CAD build for the part. Positions are in the model's coordinates, mm. A direction names the side the tool comes from. Round coordinates to 2 decimals unless told otherwise and drop trailing zeros. Loops run counter-clockwise (first coordinate to the right, second up) from the corner with the lowest first, then second, coordinate; pieces in that order, holes last.
Autodesk Inventor part; units mm, degrees
ref_plane "YZ Plane" through (0, 0, 0) normal (1, 0, 0) x (0, 1, 0)
ref_plane "XZ Plane" through (0, 0, 0) normal (0, 1, 0) x (-1, 0, 0)
ref_plane "XY Plane" through (0, 0, 0) normal (0, 0, 1) x (1, 0, 0)
sketch "Sketch1" plane through (0, 0, 0) normal (0, 0, 1) x (1, 0, 0)
  line L0 (-14, 17.1738) -> (14, 17.1738)
  line L1 (14, 17.1738) -> (14, -17.1738)
  line L2 (14, -32.8262) -> (-14, -32.8262)
  line L3 (-14, -32.8262) -> (-14, -17.1738)
  arc A0 (-14, -17.1738) -> (14, -17.1738) centre (0, -32.8262) ccw
  line L4 (-14, -17.1738) -> (-14, 17.1738)
  line L5 (14, -17.1738) -> (14, -32.8262)
  point P0 (0, 0)
  point P1 (0, 17.1738)
  point P2 (14, 0)
  dimension "d0" = 42
  dimension "d1" = 50
  dimension "d4" = 28
extrude "Extrusion1" add sketch "Sketch1" along normal blind 3
sketch "Sketch2" plane through (0, 0, 3) normal (0, 0, 1) x (1, 0, 0)
  line L0 (14, -17.1738) -> (14, 17.1738)
  line L1 (14, 17.1738) -> (-14, 17.1738) construction
  line L2 (-14, 17.1738) -> (-14, -17.1738) construction
  arc A0 (-14, -17.1738) -> (14, -17.1738) centre (0, -32.8262) ccw
  circle A1 centre (0, -32.8262) radius 16.75
  circle A2 centre (0, -32.8262) radius 21
  line L3 (-14, -2.8262) -> (14, -2.8262)
  line L4 (14, -17.1738) -> (14, 17.1738) construction
  line L5 (-14, 17.1738) -> (-14, -17.1738)
  line L6 (-14, -2.8262) -> (-14, -17.1738)
  line L7 (-9, -2.8262) -> (-9, -13.8526)
  line L8 (14, -2.8262) -> (14, -17.1738)
  line L9 (9, -13.8526) -> (9, -2.8262)
  arc A3 (-14, -17.1738) -> (14, -17.1738) centre (0, -32.8262) ccw
  line L10 (14, -2.8262) -> (14, -17.1738)
  point P0 (0, 0)
  dimension "d5" = 33.5
  dimension "d6" = 20
  dimension "d7" = 5
  dimension "d8" = 5
extrude "Extrusion2" add sketch "Sketch2" along normal blind 3 contours A2 L9 L3 L0 | A0 A2 | L5 L3 L7 A2
sketch "Sketch3" plane through (0, 0, 3) normal (0, 0, 1) x (1, 0, 0)
  circle A0 centre (0, -32.8262) radius 16.75
  circle A1 centre (0, -32.8262) radius 5
  line L0 (9, -2.8262) -> (14, -2.8262)
  line L1 (14, -2.8262) -> (14, 17.1738)
  line L2 (14, 17.1738) -> (-14, 17.1738)
  line L3 (-14, 17.1738) -> (-14, -2.8262)
  line L4 (-14, -2.8262) -> (-9, -2.8262)
  line L5 (-9, -2.8262) -> (-9, -13.8526)
  arc A2 (9, -13.8526) -> (-9, -13.8526) centre (0, -32.8262) ccw
  line L6 (9, -13.8526) -> (9, -2.8262)
  circle A3 centre (-6, 7.1738) radius 2.1
  circle A4 centre (6, 7.1738) radius 2.1
  line L7 (-6, 7.1738) -> (6, 7.1738) construction
  point P0 (0, 0)
  point P1 (0, 7.1738)
  dimension "d11" = 10
  dimension "d12" = 4.2
  dimension "d13" = 12
  dimension "d14" = 10
extrude "Extrusion3" cut sketch "Sketch3" against normal up to next contours A1 | A3 | A4
chamfer "Chamfer1" distance 3 angle 45 2 edges at (11.5, -2.8262, 6) (-11.5, -2.8262, 6)
fillet "Fillet1" radius 1 7 edges at (-16.75, -32.8262, 6) (0, -11.8262, 6) (0, -53.8262, 6) (-14, -11.4998, 6) (-9, -9.8392, 6) (9, -9.8392, 6) (14, -11.4998, 6)
sketch "Sketch4" plane through (0, -32.8262, 3) normal (0, 0, 1) x (1, 0, 0)
  circle A0 centre (0, 0) radius 5
  circle A1 centre (8.4853, 8.4853) radius 1.65
  line L0 (0, 0) -> (8.4853, 8.4853) construction
  line L1 (0, 0) -> (0, 12.1192) construction
  line L2 (0, 0) -> (-12.1192, 0) construction
  circle A2 centre (-8.4853, 8.4853) radius 1.65
  line L3 (0, 0) -> (0, -12.1192) construction
  circle A3 centre (-8.4853, -8.4853) radius 1.65
  line L4 (0, 0) -> (12.1192, 0) construction
  circle A4 centre (8.4853, -8.4853) radius 1.65
  point P0 (0, 32.8262)
  dimension "d21" = 45
  dimension "d22" = 3.3
  dimension "d23" = 12
  dimension "d26" = 360
extrude "Extrusion4" cut sketch "Sketch4" against normal up to next contours A1 | A2 | A3 | A4
fillet "Fillet2" radius 4 2 edges at (-14, 17.1738, 1.5) (14, 17.1738, 1.5)
equation "\"d8\" = d7"
properties part number "holder-LMF8LUU-z-axis"
Item 1: Cut at A-A (x = 0). List the corners of the cut face in (y, z).
Verdict:
outline: (-53.83, 0) - (-37.83, 0) - (-37.83, 3) - (-49.58, 3) - (-49.58, 5) arc R1 ccw to (-50.58, 6) - (-52.83, 6) arc R1 ccw to (-53.83, 5) - close; (-27.83, 0) - (17.17, 0) - (17.17, 3) - (-11.83, 3) - (-11.83, 5) arc R1 ccw to (-12.83, 6) - (-15.08, 6) arc R1 ccw to (-16.08, 5) - (-16.08, 3) - (-27.83, 3) - close
Item 2: Flat gauge pins, fed straight in: P1, Ø5.5, axis at x = -8.49, y = -24.34, coming from the +Z side; P2, Ø0.6, axis at y = -7, z = 4, coming from the +X side; P3, Ø1, axis at x = 14, z = 1, coming from the -Y side. Where does each tip first touch, or does it go through?
Verdict:
P1: stops at z = 3
P2: stops at x = 14
P3: stops at y = -48.91
Item 3: Wall check: L1, parallel to Y at x = 7, z = 1; L2, parallel to Z at x = -6, y = -35; L3, parallel to X at y = -31.5, z = 1.5. Give the ranges that are in metal, low to high.
Verdict:
L1: y = -52.63 to -42.03, -40.59 to -25.06, -23.62 to 5.33, 9.02 to 17.17
L2: z = 0 to 3
L3: x = -20.96 to -4.82, 4.82 to 20.96
Item 4: Mould opens along X. For faces 6 (the flat face through (0, -18, 0)), 7 (the cylindrical face through (9.247, -25.805, 1.521)), 8 (the cylindrical face through (12.86, 15.97, 1.52)) say: released by +X, released by -X, zero draft, split by the parting line, or undercut.
Verdict:
face 6: zero draft
face 7: undercut
face 8: released by +X
Item 5: Cut at B-B (z = 4.25). List the corners of the cut face in (x, y).
Verdict:
outline: (-14, -17.17) arc R21 ccw (long way) to (14, -17.17) - (14, -4.08) - (9, -4.08) - (9, -13.85) arc R21 ccw to (-9, -13.85) - (-9, -4.08) - (-14, -4.08) - close; hole circle Ø33.5 at (0, -32.83)
Item 6: 3-axis set-ups, long thin cutter, end or side, ignore diameter. For faces 1 (the flat face through (-9, -8, 4)), 2 (the flat face through (14, -5, 2)), 3 (the flat face through (-3, -15, 6)), 4 (the cylindrical face through (-3.631, -16.475, 3.986)), 5 (the cylindrical face through (-7.724, -25.805, 1.521)): which of +Z, -Z, +X, -X, +Y, -Y reach the whole face in a straight line?
Verdict:
face 1: +Z, +Y
face 2: +Z, -Z, +X, +Y
face 3: +Z, +X, -X, +Y, -Y
face 4: +Z
face 5: +Z, -Z
Item 7: Cut at C-C (y = 0.5). List the corners of the cut face in (x, z).
Verdict:
outline: (-14, 0) - (14, 0) - (14, 3) - (-14, 3) - close
